Check sheet for the modelled part. Datum: model origin and axes. Units: mm. A direction names the side the tool comes from. Round coordinates to 2 decimals unless told otherwise and drop trailing zeros. Loops run counter-clockwise (first coordinate to the right, second up) from the corner with the lowest first, then second, coordinate; pieces in that order, holes last. Notation, with made-up numbers: (-13.5, -36) - (15.5, -36) arc R15 ccw to (15.5, -27) - close; hole circle Ø6 at (-20, 77.25). An arc over 180 degrees is marked (long way). Answer in a Markdown table with one row per item. Add a question column.
(1) Cross-section at C-C on x = 660.4. Enter the section's corners in (y, z), then the cut area to 3 significant figures.
(2) Mould release check, pull along X, two halves, no side actions. Record for faces 1 (the flat face through (0, 64, 22)), 2 (the flat face through (63.5, 42, 22)), 3 (the flat face through (698.7, 126.8, 21.9)): +X half, -X half, draft (parallel to the pull), parting line (faces both ways), or undercut.
(3) Cross-section at D-D on x = 114. Enter the section's corners in (y, z).
(4) Access from +Z, -Z, +X, -X, +Y, -Y to the whole of each face (thin tool, end or side, straight path). Record for faces 4 (the flat face through (360, 139.7, 22)), 5 (the flat face through (647.7, 41, 22)).
(5) Cross-section at A-A on z = 24.5. Enter the section's corners in (x, y), then the cut area to 3 significant figures.
(6) Cross-section at B-B on y = 21.5. Enter the section's corners in (x, z).
(7) Thickness scan on line 1 along X through (y, z) = (76, 12); line 2 along X through (y, z) = (91.5, 29.5); line 3 along X through (y, z) = (121.5, 42). Record the ranges inside material, lowest first.
(8) Gauge pin test, flat end, axial feed: pin 1 (5 mm diameter, centred on y = 122.5, z = 16.5, fed in from +X). Record the tip position at first contact, or that the pin passes through.
from build123d import *

# Parameters (mm, degrees)
F1_DEPTH = 44.45
F2_SIZE  = 12.7


with BuildPart() as f1:
    # F0 (on Top) → F1 (new body)
    with BuildSketch(Plane.XY):
        with BuildLine():
            ThreePointArc((38.1, 82.55), (50.8, 95.25), (63.5, 82.55))
            Line((63.5, 82.55), (63.5, 0))
            Line((63.5, 0), (105.023582, 0))
            Line((105.023582, 0), (355.6, 0))
            Line((355.6, 0), (606.176418, 0))
            Line((606.176418, 0), (647.7, 0))
            Line((647.7, 0), (647.7, 82.55))
            ThreePointArc((647.7, 82.55), (660.4, 95.25), (673.1, 82.55))
            Line((673.1, 82.55), (673.1, 0))
            Line((673.1, 0), (698.5, 0))
            ThreePointArc((698.5, 0), (702.219744, 8.980256), (711.2, 12.7))
            Line((711.2, 12.7), (711.2, 114.3))
            Line((711.2, 114.3), (685.8, 139.7))
            Line((685.8, 139.7), (355.6, 139.7))
            Line((355.6, 139.7), (25.4, 139.7))
            Line((25.4, 139.7), (0, 114.3))
            Line((0, 114.3), (0, 12.7))
            ThreePointArc((0, 12.7), (8.980256, 8.980256), (12.7, 0))
            Line((12.7, 0), (38.1, 0))
            Line((38.1, 0), (38.1, 82.55))
        make_face()
    extrude(amount=F1_DEPTH)

    # F2
    f2_edges = [f1.edges().sort_by_distance(p)[0] for p in [
        (355.6, 139.7, 44.45),
        (355.6, 139.7, 0),
    ]]
    chamfer(f2_edges, length=F2_SIZE)


solid = f1.part
Answers:
| question | item | result |
|---|---|---|
| 1 | outline | (95.25, 0) - (127, 0) - (139.7, 12.7) - (139.7, 31.75) - (127, 44.45) - (95.25, 44.45) - close |
| 1 | area | 1,810 mm^2 |
| 2 | face 1 | -X half |
| 2 | face 2 | undercut |
| 2 | face 3 | +X half |
| 3 | outline | (0, 0) - (127, 0) - (139.7, 12.7) - (139.7, 31.75) - (127, 44.45) - (0, 44.45) - close |
| 4 | face 4 | +Z, -Z, +X, -X, +Y |
| 4 | face 5 | +Z, -Z, -Y |
| 5 | outline | (0, 12.7) arc R12.7 cw to (12.7, 0) - (38.1, 0) - (38.1, 82.55) arc R12.7 cw to (63.5, 82.55) - (63.5, 0) - (647.7, 0) - (647.7, 82.55) arc R12.7 cw to (673.1, 82.55) - (673.1, 0) - (698.5, 0) arc R12.7 cw to (711.2, 12.7) - (711.2, 114.3) - (685.8, 139.7) - (25.4, 139.7) - (0, 114.3) - close |
| 5 | area | 93,800 mm^2 |
| 6 | outline | (0, 0) - (38.1, 0) - (38.1, 44.45) - (0, 44.45) - close; (63.5, 0) - (647.7, 0) - (647.7, 44.45) - (63.5, 44.45) - close; (673.1, 0) - (711.2, 0) - (711.2, 44.45) - (673.1, 44.45) - close |
| 7 | line 1 | x = 0 to 38.1, 63.5 to 647.7, 673.1 to 711.2 |
| 7 | line 2 | x = 0 to 41.79, 59.81 to 651.39, 669.41 to 711.2 |
| 7 | line 3 | x = 7.2 to 704 |
| 8 | pin 1 | stops at x = 705.5 |
